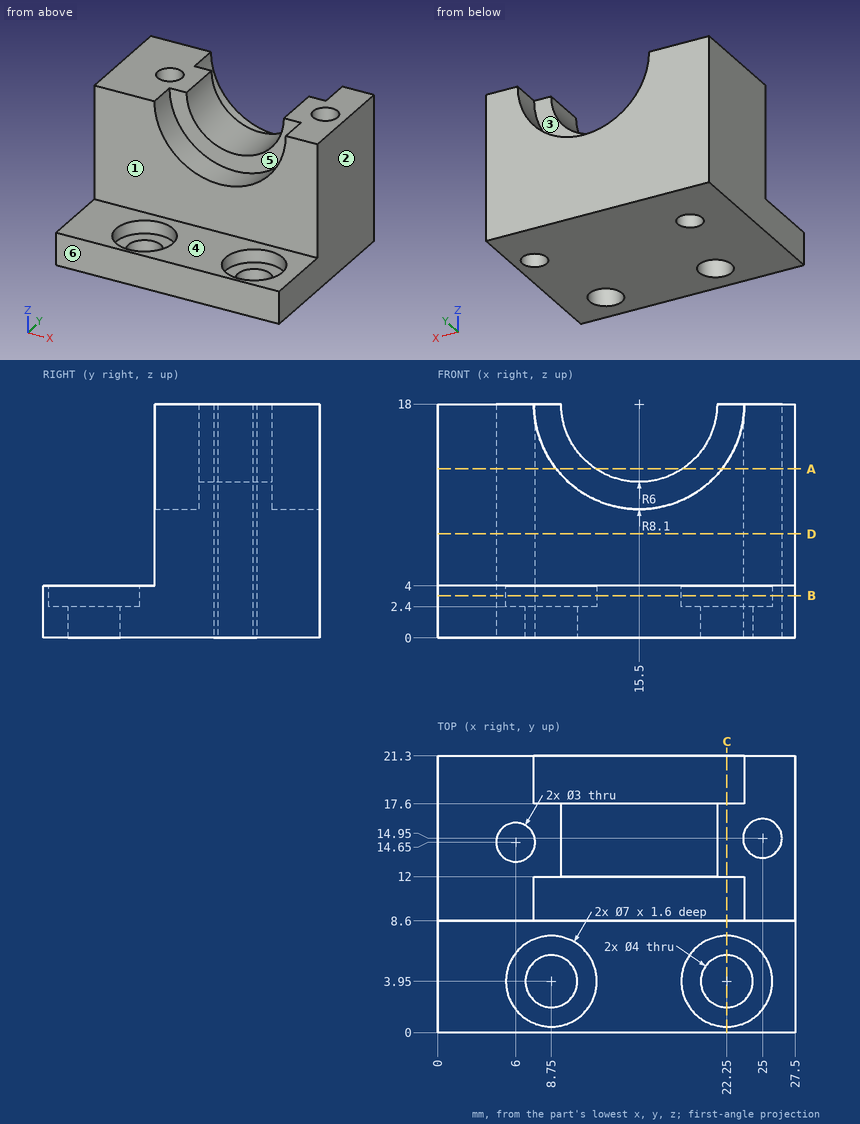
Source: three-view drawing plus pictorial views. Frame: mm from the lowest corner of the part. A direction names the side the tool comes from. Round coordinates to 2 decimals unless told otherwise and drop trailing zeros. Loops run counter-clockwise (first coordinate to the right, second up) from the corner with the lowest first, then second, coordinate; pieces in that order, holes last.
Q1. Pin query (flat end, axial travel): P1, Ø9.5, axis at x = 19.5, y = 3, coming from the +Z side; P2, Ø1.8, axis at x = 6, y = 14.65, coming from the -Z side; P3, Ø4.5, axis at x = 22.25, y = 3.95, coming from the +Z side; P4, Ø1, axis at x = 18.5, z = 12, coming from the +Y side. Return the tip coordinate at first contact, or that it passes through.
Q2. Section C-C on x = 22.25. Return loops of the section in (y, z), plus the area to 3 significant figures.
Q3. Section A-A on z = 13. Return loops of the section in (x, y).
Q4. Pull-direction query (X, two-part tool) for the marked faces 1, 2 and 3; classes: released by +X, released by -X, zero draft, split by the parting line, or undercut.
Q5. Section B-B on z = 3.25. Return loops of the section in (x, y).
Q6. Section D-D on z = 8. Return loops of the section in (x, y).
Q7. Material intervals for L1, parallel to Y at x = 8.75, z = 2.8; L2, parallel to X at y = 14.75, z = 2.25; L3, parallel to Y at x = 22.25, z = 1.55, sorted ascending.
Q8. Access query for the marked faces 4, 5 and 6. Directions: +Z, -Z, +X, -X, +Y, -Y. A direction counts if a zero-diameter tool reaches every point of the face in a straight line with its end or side. Return the directions, or none.
Evaluation:
1. P1: stops at z = 4
1. P2: passes through
1. P3: stops at z = 2.4
1. P4: stops at y = 17.6
2. outline: (0, 0) - (1.95, 0) - (1.95, 2.4) - (0.45, 2.4) - (0.45, 4) - (0, 4) - close; (5.95, 0) - (21.3, 0) - (21.3, 13.52) - (17.6, 13.52) - (17.6, 18) - (12, 18) - (12, 13.52) - (8.6, 13.52) - (8.6, 4) - (7.45, 4) - (7.45, 2.4) - (5.95, 2.4) - close
2. area: 210 mm2
3. outline: (0, 8.6) - (9.13, 8.6) - (9.13, 12) - (12.18, 12) - (12.18, 17.6) - (9.13, 17.6) - (9.13, 21.3) - (0, 21.3) - close; (18.82, 12) - (21.87, 12) - (21.87, 8.6) - (27.5, 8.6) - (27.5, 21.3) - (21.87, 21.3) - (21.87, 17.6) - (18.82, 17.6) - close; hole circle Ø3 at (6, 14.65); hole circle Ø3 at (25, 14.95)
4. face 1: zero draft
4. face 2: released by +X
4. face 3: undercut
5. outline: (0, 0) - (27.5, 0) - (27.5, 21.3) - (0, 21.3) - close; hole circle Ø3 at (6, 14.65); hole circle Ø7 at (8.75, 3.95); hole circle Ø7 at (22.25, 3.95); hole circle Ø3 at (25, 14.95)
6. outline: (0, 8.6) - (27.5, 8.6) - (27.5, 21.3) - (0, 21.3) - close; hole circle Ø3 at (6, 14.65); hole circle Ø3 at (25, 14.95)
7. L1: y = 0 to 0.45, 7.45 to 21.3
7. L2: x = 0 to 4.5, 7.5 to 23.51, 26.49 to 27.5
7. L3: y = 0 to 1.95, 5.95 to 21.3
8. face 4: +Z, +X, -X, -Y
8. face 5: +Z, -Y
8. face 6: +Z, -Z, +X, -X, -Y
